Here's how the part is built. I have some questions about the finished solid (model axes, mm). Face numbers are marked on the shaded views. Coordinates: 2 decimals unless noted, no trailing zeros. Write each loop counter-clockwise with the first axis right and the second up, starting at its lowest first coordinate (ties: lowest second). Pieces come first, ordered by that corner, then holes. Notation, with made-up numbers: M 62,3.25 L 76,3.25 A30 cw 76,37.25 Z; hole C 8,69 d3. An arc over 180 degrees is marked long. Use a Markdown table: item, result.
```python
from build123d import *

# Parameters (mm, degrees)
F0_W     = 37
F0_H     = 15
F1_DEPTH = 62
F3_DEPTH = 62.001
F4_DEPTH = 2


with BuildPart() as f1:
    # F0 (on Top) → F1 (new body)
    with BuildSketch(Plane.XY):
        with Locations((18.5, 7.5)):
            Rectangle(F0_W, F0_H)
    extrude(amount=F1_DEPTH)

    # F2 (on face) → F3 (cut, through all)
    with BuildSketch(Plane(origin=(0, 0, 0), x_dir=(1, 0, 0), z_dir=(0, 0, -1))):
        with BuildLine():
            Line((13.3, 0), (3.7, 0))
            ThreePointArc((3.7, 0), (8.5, -4.8), (13.3, 0))
        make_face()
        with BuildLine():
            Line((33.3, 0), (23.7, 0))
            ThreePointArc((23.7, 0), (28.5, -4.8), (33.3, 0))
        make_face()
    extrude(amount=-F3_DEPTH, mode=Mode.SUBTRACT)

    # F4 (cut): a face of the model
    f4_faces = [f1.faces().sort_by_distance(p)[0] for p in [
        (18.5, 15, 31),
    ]]
    extrude(f4_faces, amount=-F4_DEPTH, mode=Mode.SUBTRACT)


solid = f1.part
```
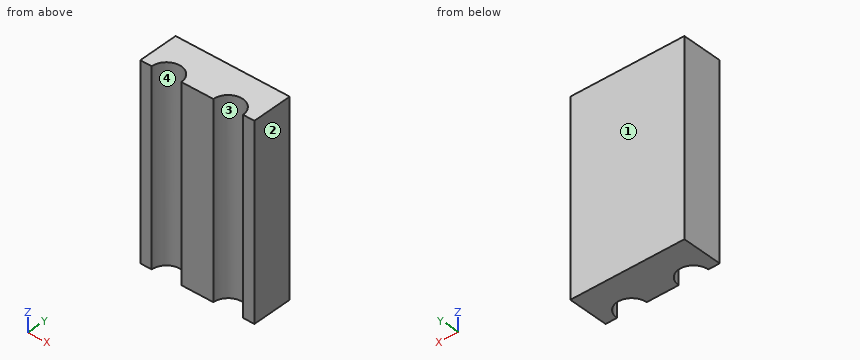
1. Suppose I cut it at B-B on z = 26. Write out the boundary of the cut face in (x, y).
Answers follow:
| item | result |
|---|---|
| outline | M 0,0 L 3.7,0 A4.8 cw 13.3,0 L 23.7,0 A4.8 cw 33.3,0 L 37,0 L 37,13 L 0,13 Z |
2. Suppose I cut it at C-C on x = 28.5. Write out the boundary of the cut face in (y, z).
Answers follow:
| item | result |
|---|---|
| outline | M 4.8,0 L 13,0 L 13,62 L 4.8,62 Z |
3. I need wall thicknesses on probe 1 along X at (y, z) = (0.75, 19); probe 2 along X at (y, z) = (2.5, 56); probe 3 along Y at (x, z) = (7, 32.5). Which ranges of each line are inside material? Lowest first, please.
Answers follow:
| item | result |
|---|---|
| probe 1 | x = 0 to 3.76, 13.24 to 23.76, 33.24 to 37 |
| probe 2 | x = 0 to 4.4, 12.6 to 24.4, 32.6 to 37 |
| probe 3 | y = 4.56 to 13 |
4. Will this pin go through, and if not, where does the flat tip stop? pin 1 Ø2 at (x, z) = (9, 37) entering from -Y.
Answers follow:
| item | result |
|---|---|
| pin 1 | stops at y = 4.56 |
5. We'd pull the mould along X, two halves only. Please class the marked faces 1, 2, 3 and 4: +X half, -X half, draft (parallel to the pull), parting line (faces both ways), or undercut.
Answers follow:
| item | result |
|---|---|
| face 1 | draft |
| face 2 | +X half |
| face 3 | undercut |
| face 4 | undercut |
6. Suppose I cut it at A-A on y = 3.5. Write out the boundary of the cut face in (x, z), and give its area (3 significant figures).
Answers follow:
| item | result |
|---|---|
| outline | M 0,0 L 5.22,0 L 5.22,62 L 0,62 Z; M 11.78,0 L 25.22,0 L 25.22,62 L 11.78,62 Z; M 31.78,0 L 37,0 L 37,62 L 31.78,62 Z |
| area | 1,480 mm2 |
